Model file for the job. Use its own axes, mm. A direction names the side the tool comes from. Coordinates: 2 decimals unless noted, no trailing zeros. Order: outer loops, then holes, each group sorted by start corner. A loop starts at its lowest first (then second) coordinate and runs counter-clockwise, first axis right, second up. Notation, with made-up numbers: (6.25, -38) -> (50.25, -38) arc R27 ccw to (50.25, -16) -> close; hole circle Ø11 at (-29.75, 11.5). An arc over 180 degrees is marked (long way). Use CSV: the item, a comma, the result in double quotes. Start each with the question number.
(1) Tool access for faces 5 (the cylindrical face through (602.35, -178.38, -257.28)), 6 (the cylindrical face through (629.617, -195.874, 249.142)), 7 (the flat face through (-455, -40, -3)), 8 (the flat face through (-430, -86, 245)), 9 (the flat face through (600, -27, 4)): list every direction of +Z, -Z, +X, -X, +Y, -Y with a clear straight run to the whole face (end or side of a thin tool).
(2) Cut at B-B on x = 296.5. Write the cut outline in (y, z).
(3) Probe L1, parallel to Z at x = 338, y = -165.5; L2, parallel to Y at x = -334, z = -229.5; L3, parallel to X at y = -26, z = 97. List the from-to ranges inside material, lowest first.
(4) Pull direction X, two halves, no side cores. Call faces 1 (the flat face through (586, -205, 254)), 2 (the flat face through (-480, -27, 4)), 3 (the flat face through (53, -150, 220)), 4 (the flat face through (53, -40, -245)): pulls with the +X half, pulls with the -X half, needs draft (parallel to the pull), parting line crosses it, or undercut.
(5) Cut at C-C on y = -159. Write the cut outline in (x, z), plus the area to 3 significant figures.
(6) Pin check, flat tips, straight feed: pin 1 Ø25 at (y, z) = (-82, 247) entering from +X; pin 2 Ø1 at (x, z) = (363, 222.5) entering from -Y; pin 3 Ø15 at (x, z) = (-464.5, 80) entering from +Y; pin 4 Ø20 at (x, y) = (231, -145.5) entering from -Z. Stop position of each tip, or through.
(7) Cut at A-A on y = -57.5. Write the cut outline in (x, z).
```python
from build123d import *

# Parameters (mm, degrees)
SKETCH_1_W             = 1080
SKETCH_1_H             = 540
SKETCH_1_W_2           = 980
SKETCH_1_H_2           = 440
EXTRUDE_1_DEPTH        = 170
SKETCH_2_W             = 980
SKETCH_2_H             = 90
CUT_EXTRUDE_1_DEPTH    = 825.924238946
SKETCH_3_W             = 440
SKETCH_3_H             = 90
CUT_EXTRUDE_2_DEPTH    = 1127.143862923
FOUR_START             = -187
SKETCH_6_R             = 45
FOUR_BASE_PADS_DEPTH   = 18
FOUR_BASE_PADS_2_DEPTH = 18
FOUR_BASE_PADS_3_DEPTH = 18
FOUR_BASE_PADS_4_DEPTH = 18
FOUR_START_2           = -170
SKETCH_7_R             = 17.5
FOUR_FOOT_STEMS_DEPTH  = 17


with BuildPart() as part:
    # 草图1 → 拉伸-薄壁1 (new body)
    with BuildSketch(Plane(origin=(0, 0, 0), x_dir=(1, 0, 0), z_dir=(0, 1, 0))):
        with Locations((60, 0)):
            Rectangle(SKETCH_1_W, SKETCH_1_H)
        with Locations((60, 0)):
            Rectangle(SKETCH_1_W_2, SKETCH_1_H_2, mode=Mode.SUBTRACT)
    extrude(amount=-EXTRUDE_1_DEPTH)

    # 草图2 → 切除-拉伸1 (cut, through all)
    with BuildSketch(Plane.XY.offset(270)):
        with Locations((60, -85)):
            Rectangle(SKETCH_2_W, SKETCH_2_H)
    extrude(amount=-CUT_EXTRUDE_1_DEPTH, mode=Mode.SUBTRACT)

    # 草图3 → 切除-拉伸2 (cut, through all)
    with BuildSketch(Plane.ZY.offset(480)):
        with Locations((0, -85)):
            Rectangle(SKETCH_3_W, SKETCH_3_H)
    extrude(amount=-CUT_EXTRUDE_2_DEPTH, mode=Mode.SUBTRACT)



with BuildPart() as body_2:
    # 草图6 → Four Base Pads (new body)
    with BuildSketch(Plane(origin=(0, 0, 0), x_dir=(1, 0, 0), z_dir=(0, 1, 0)).offset(FOUR_START)):
        with Locations(Location((-465, -255, 0), (0, 0, 270))):
            Circle(SKETCH_6_R)
    extrude(amount=-FOUR_BASE_PADS_DEPTH)


with BuildPart() as body_3:
    # 草图6 → Four Base Pads 2 (new body)
    with BuildSketch(Plane(origin=(0, 0, 0), x_dir=(1, 0, 0), z_dir=(0, 1, 0)).offset(FOUR_START)):
        with Locations(Location((-465, 255, 0), (0, 0, 270))):
            Circle(SKETCH_6_R)
    extrude(amount=-FOUR_BASE_PADS_2_DEPTH)


with BuildPart() as body_4:
    # 草图6 → Four Base Pads 3 (new body)
    with BuildSketch(Plane(origin=(0, 0, 0), x_dir=(1, 0, 0), z_dir=(0, 1, 0)).offset(FOUR_START)):
        with Locations(Location((585, -255, 0), (0, 0, 270))):
            Circle(SKETCH_6_R)
    extrude(amount=-FOUR_BASE_PADS_3_DEPTH)


with BuildPart() as body_5:
    # 草图6 → Four Base Pads 4 (new body)
    with BuildSketch(Plane(origin=(0, 0, 0), x_dir=(1, 0, 0), z_dir=(0, 1, 0)).offset(FOUR_START)):
        with Locations(Location((585, 255, 0), (0, 0, 270))):
            Circle(SKETCH_6_R)
    extrude(amount=-FOUR_BASE_PADS_4_DEPTH)


with BuildPart() as part_1:
    add(part.part)

    add(body_2.part)  # Four Foot Stems merges body 2

    add(body_3.part)  # Four Foot Stems merges body 3

    add(body_4.part)  # Four Foot Stems merges body 4

    add(body_5.part)  # Four Foot Stems merges body 5
    # 草图7 → Four Foot Stems (add)
    with BuildSketch(Plane(origin=(0, 0, 0), x_dir=(1, 0, 0), z_dir=(0, 1, 0)).offset(FOUR_START_2)):
        with Locations(Location((-465, -255, 0), (0, 0, 270))):
            Circle(SKETCH_7_R)
        with Locations(Location((-465, 255, 0), (0, 0, 270))):
            Circle(SKETCH_7_R)
        with Locations(Location((585, -255, 0), (0, 0, 270))):
            Circle(SKETCH_7_R)
        with Locations(Location((585, 255, 0), (0, 0, 270))):
            Circle(SKETCH_7_R)
    extrude(amount=-FOUR_FOOT_STEMS_DEPTH)


solid = part_1.part
```
Outcome:
1,face 5,"none"
1,face 6,"-Y"
1,face 7,"+X, -X"
1,face 8,"+Z, -Z"
1,face 9,"+Z, -Z, +X, +Y"
2,outline,"(-170, -270) -> (-130, -270) -> (-130, -220) -> (-170, -220) -> close; (-170, 220) -> (-130, 220) -> (-130, 270) -> (-170, 270) -> close; (-40, -270) -> (0, -270) -> (0, -220) -> (-40, -220) -> close; (-40, 220) -> (0, 220) -> (0, 270) -> (-40, 270) -> close"
3,L1,"-270 to -220, 220 to 270"
3,L2,"-170 to -130, -40 to 0"
3,L3,"-480 to -430, 550 to 600"
4,face 1,"needs draft"
4,face 2,"pulls with the -X half"
4,face 3,"undercut"
4,face 4,"undercut"
5,outline,"(-480, -270) -> (600, -270) -> (600, 270) -> (-480, 270) -> close; hole (-430, -220) -> (550, -220) -> (550, 220) -> (-430, 220) -> close"
5,area,"152,000 mm2"
6,pin 1,"x = 600"
6,pin 2,"y = -170"
6,pin 3,"y = 0"
6,pin 4,"z = -270"
7,outline,"(-480, -270) -> (-430, -270) -> (-430, -220) -> (-480, -220) -> close; (-480, 220) -> (-430, 220) -> (-430, 270) -> (-480, 270) -> close; (550, -270) -> (600, -270) -> (600, -220) -> (550, -220) -> close; (550, 220) -> (600, 220) -> (600, 270) -> (550, 270) -> close"
